Part print with two shaded views. Sizes in mm from the minimum x, y, z corner. Give positions to 0.01 mm unless a question says otherwise; leave off trailing zeros. Write each loop counter-clockwise with the first axis right and the second up, starting at its lowest first coordinate (ties: lowest second). Pieces come first, ordered by that corner, then holes. Notation, with made-up numbers: (82, 20.5) - (108, 20.5) arc R20 cw to (108, 30.5) - close; hole circle Ø6 at (55.5, -38.75). An arc over 180 degrees is marked (long way). Answer as a JSON object with one key per item and string values.
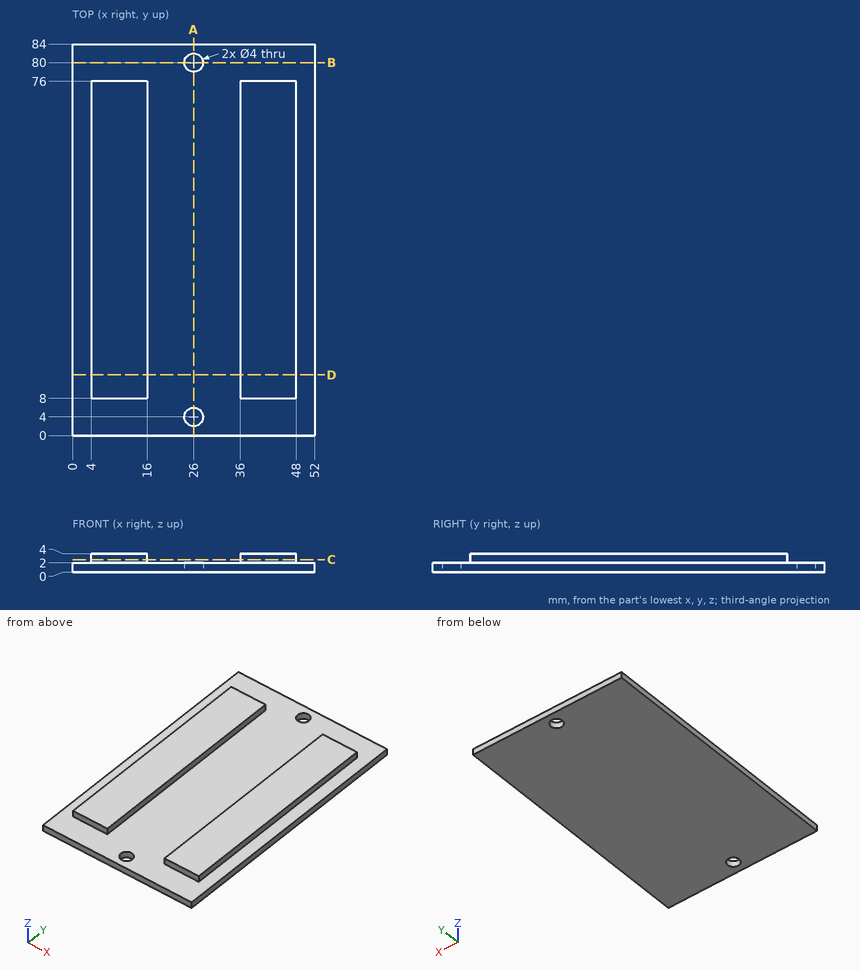
(1) Saw through at A-A, the plane x = 26. Give the cut face in (y, z), and give its area (3 significant figures).
Answer key:
{"outline": "(0, 0) - (2, 0) - (2, 2) - (0, 2) - close; (6, 0) - (78, 0) - (78, 2) - (6, 2) - close; (82, 0) - (84, 0) - (84, 2) - (82, 2) - close", "area": "152 mm²"}
(2) Saw through at C-C, the plane z = 2.7. Give the cut face in (x, y).
Answer key:
{"outline": "(4, 8) - (16, 8) - (16, 76) - (4, 76) - close; (36, 8) - (48, 8) - (48, 76) - (36, 76) - close"}
(3) Flat gauge pins, fed straight in: P1, Ø3.5, axis at x = 26, y = 80, coming from the -Z side; P2, Ø12, axis at x = 27, y = 30, coming from the -Z side; P3, Ø0.6, axis at y = 28.5, z = 2.5, coming from the -X side; P4, Ø2, axis at x = 44.5, z = 3.5, coming from the +Y side. Where does each tip first touch, or does it go through?
Answer key:
{"P1": "passes through", "P2": "stops at z = 0", "P3": "stops at x = 4", "P4": "stops at y = 76"}
(4) Saw through at D-D, the plane y = 13. Give the cut face in (x, z).
Answer key:
{"outline": "(0, 0) - (52, 0) - (52, 2) - (48, 2) - (48, 4) - (36, 4) - (36, 2) - (16, 2) - (16, 4) - (4, 4) - (4, 2) - (0, 2) - close"}
(5) Saw through at B-B, the plane y = 80. Give the cut face in (x, z).
Answer key:
{"outline": "(0, 0) - (24, 0) - (24, 2) - (0, 2) - close; (28, 0) - (52, 0) - (52, 2) - (28, 2) - close"}
(6) Probe L1, parallel to Y at x = 26, z = 1.9; L2, parallel to X at y = 63.5, z = 2.35; L3, parallel to X at y = 80, z = 0.5. List the from-to ranges inside material, lowest first. Write a range as [from, to].
Answer key:
{"L1": "y = [0, 2], [6, 78], [82, 84]", "L2": "x = [4, 16], [36, 48]", "L3": "x = [0, 24], [28, 52]"}
